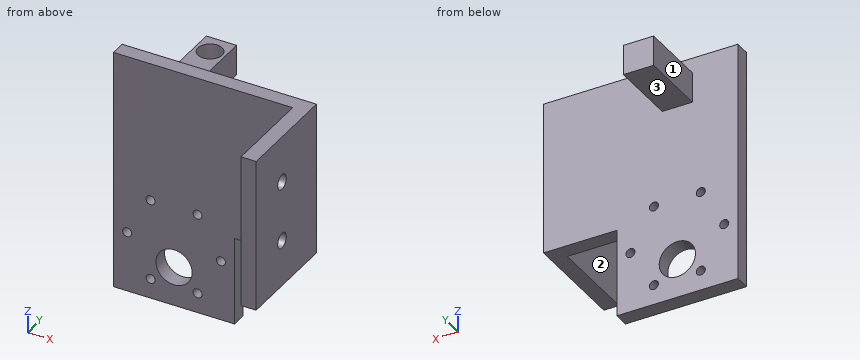
from build123d import *

# Parameters (mm, degrees)
SKETCH3_W           = 40
SKETCH3_H           = 80
BOSS_EXTRUDE1_DEPTH = 5
SKETCH1_R           = 1.5
SKETCH1_R_2         = 6
CUT_EXTRUDE3_DEPTH  = 64.442887702
SKETCH4_W           = 10
SKETCH4_H           = 10
BOSS_EXTRUDE2_DEPTH = 22.5
SKETCH5_R           = 4
CUT_EXTRUDE4_DEPTH  = 8
SKETCH6_W           = 50.8
SKETCH6_H           = 5
BOSS_EXTRUDE3_DEPTH = 24.225
SKETCH8_W           = 5
SKETCH8_H           = 50.8
BOSS_EXTRUDE4_DEPTH = 30
SKETCH9_R           = 2.5
CUT_EXTRUDE5_DEPTH  = 5


with BuildPart() as part:
    # Sketch3 → Boss-Extrude1 (new body)
    with BuildSketch(Plane(origin=(0, 0, 0), x_dir=(1, 0, 0), z_dir=(0, 1, 0))):
        with Locations((0, -20)):
            Rectangle(SKETCH3_W, SKETCH3_H)
    extrude(amount=BOSS_EXTRUDE1_DEPTH)

    # Sketch1 → Cut-Extrude3 (cut, through all)
    with BuildSketch(Plane(origin=(0, 0, 0), x_dir=(1, 0, 0), z_dir=(0, 1, 0))):
        with Locations(Location((-15.5, 0, 0), (0, 0, 270))):
            Circle(SKETCH1_R)
        with Locations(Location((-7.75, 13.423393759, 0), (0, 0, 270))):
            Circle(SKETCH1_R)
        with Locations(Location((7.75, 13.423393759, 0), (0, 0, 270))):
            Circle(SKETCH1_R)
        with Locations(Location((15.5, 0, 0), (0, 0, 270))):
            Circle(SKETCH1_R)
        with Locations(Location((7.75, -13.423393759, 0), (0, 0, 270))):
            Circle(SKETCH1_R)
        with Locations(Location((-7.75, -13.423393759, 0), (0, 0, 270))):
            Circle(SKETCH1_R)
        with Locations(Location((0, 7, 0), (0, 0, 270))):
            Circle(SKETCH1_R_2)
    extrude(amount=CUT_EXTRUDE3_DEPTH, mode=Mode.SUBTRACT)

    # Sketch4 → Boss-Extrude2 (add)
    with BuildSketch(Plane(origin=(0, 5, 0), x_dir=(1, 0, 0), z_dir=(0, 1, 0))):
        with Locations((0, -50)):
            Rectangle(SKETCH4_W, SKETCH4_H)
    extrude(amount=BOSS_EXTRUDE2_DEPTH)

    # Sketch5 → Cut-Extrude4 (cut)
    with BuildSketch(Plane.XY.offset(55)):
        with Locations((0, 20.9)):
            Circle(SKETCH5_R)
    extrude(amount=-CUT_EXTRUDE4_DEPTH, mode=Mode.SUBTRACT)

    # Sketch6 → Boss-Extrude3 (add)
    with BuildSketch(Plane(origin=(20, 0, 0), x_dir=(0, 0, -1), z_dir=(1, 0, 0))):
        with Locations((-34.6, 2.5)):
            Rectangle(SKETCH6_W, SKETCH6_H)
    extrude(amount=BOSS_EXTRUDE3_DEPTH)

    # Sketch8 → Boss-Extrude4 (add)
    with BuildSketch(Plane.XZ):
        with Locations((41.725, 34.6)):
            Rectangle(SKETCH8_W, SKETCH8_H)
    extrude(amount=BOSS_EXTRUDE4_DEPTH)

    # Sketch9 → Cut-Extrude5 (cut)
    with BuildSketch(Plane(origin=(44.225, 0, 0), x_dir=(0, 0, -1), z_dir=(1, 0, 0))):
        with Locations((-44.6, -15)):
            Circle(SKETCH9_R)
        with Locations((-24.6, -15)):
            Circle(SKETCH9_R)
    extrude(amount=-CUT_EXTRUDE5_DEPTH, mode=Mode.SUBTRACT)


solid = part.part
Read the model definition and answer for the solid it produces. Units are mm, in the model's axes. Face numbers are marked on the shaded views. A direction names the side the tool comes from. Coordinates: 2 decimals unless noted, no trailing zeros. Write each loop counter-clockwise with the first axis right and the second up, starting at its lowest first coordinate (ties: lowest second). Pieces come first, ordered by that corner, then holes. Notation, with made-up numbers: (48.5, -29.5) - (68.5, -29.5) arc R24 ccw to (68.5, -17.5) - close; hole circle Ø2 at (-27, 62.5). An arc over 180 degrees is marked (long way). One line per question, with ' | ' between items.
Q1. Find section C-C, the plane x = -7.75. Write down the section's boundary in (y, z).
Result set:
outline: (0, -20) - (5, -20) - (5, -14.92) - (0, -14.92) - close; (0, -11.92) - (5, -11.92) - (5, 11.92) - (0, 11.92) - close; (0, 14.92) - (5, 14.92) - (5, 60) - (0, 60) - close
Q2. Find section A-A, the plane z = 24.6. Write down the section's boundary in (x, y) (3 decimals), plus the area to 3 significant figures.
Result set:
outline: (-20, 0) - (39.225, 0) - (39.225, -12.5) - (44.225, -12.5) - (44.225, 5) - (-20, 5) - close; (39.225, -30) - (44.225, -30) - (44.225, -17.5) - (39.225, -17.5) - close | area: 446 mm^2
Q3. Find section D-D, the plane x = 0. Write down the section's boundary in (y, z).
Result set:
outline: (0, -20) - (5, -20) - (5, -13) - (0, -13) - close; (0, -1) - (5, -1) - (5, 45) - (27.5, 45) - (27.5, 55) - (24.9, 55) - (24.9, 47) - (16.9, 47) - (16.9, 55) - (5, 55) - (5, 60) - (0, 60) - close
Q4. Consider L1, parallel to Z at x = -7.75, y = 2.4; L2, parallel to X at y = 2.15, z = 0; L3, parallel to Z at x = 0, y = 1. Determine where each line is inside the solid, lowest interval first. Write a range as [from, to].
Result set:
L1: [-20, -14.92], [-11.92, 11.92], [14.92, 60] | L2: [-20, -17], [-14, 14], [17, 20] | L3: [-20, -13], [-1, 60]
Q5. For the marked faces 1, 2 and 3, determine the directions among +Z, -Z, +X, -X, +Y, -Y from which every point of the face is accessible in a straight line to the end or side of a thin tool.
Result set:
face 1: +Z, -Z, -X, +Y | face 2: +Z, -Z, -X, -Y | face 3: -Z, +X, -X, +Y
Q6. Each of these flat-tipped pins is pushed along its axis until it touches: P1, Ø3, axis at x = 0.5, y = 17, coming from the +Z side; P2, Ø1.8, axis at x = 7.75, z = -13.42, coming from the -Y side; P3, Ø8, axis at y = 6.5, z = 3, coming from the +X side; P4, Ø15, axis at y = -12.5, z = 35.5, coming from the -X side (3 decimals). Where does it stop, or does it pass through?
Result set:
P1: z = 55 | P2: through | P3: x = 20 | P4: x = 39.225
Q7. Find section B-B, the plane z = 0. Write down the section's boundary in (x, y).
Result set:
outline: (-20, 0) - (-17, 0) - (-17, 5) - (-20, 5) - close; (-14, 0) - (14, 0) - (14, 5) - (-14, 5) - close; (17, 0) - (20, 0) - (20, 5) - (17, 5) - close
